Work out the finished part from the listing and answer in its coordinate system (mm). A direction names the side the tool comes from. Coordinates: 2 decimals unless noted, no trailing zeros. Order: outer loops, then holes, each group sorted by start corner. A loop starts at its lowest first (then second) coordinate and runs counter-clockwise, first axis right, second up. Notation, with made-up numbers: M -12.75,-29 L 46.25,-29 A17 cw 46.25,-15 Z; hole C 71.25,34.25 d8. An arc over 180 degrees is marked long. Write item = value, one per line. Start each with the question number.
Q1. Find section A-A on z = 18. Give the vertices of the cut face in (x, y), and give its area (3 significant figures).
Q2. Determine the mould class of faces 1 (the flat face through (5.735, -30.088, 12.325)), 2 (the flat face through (-5.735, 30.088, 12.325)), 3 (the flat face through (7.244, 27.181, 13.592)), 4 (the flat face through (0, 0, 0)) for opening direction X: released by +X, released by -X, zero draft, split by the parting line, or undercut.
Q3. Find section C-C on x = -27. Give the vertices of the cut face in (y, z), and give its area (3 significant figures).
Q4. Find section B-B on x = -10. Give the vertices of the cut face in (y, z), and give its area (3 significant figures).
Q5. Straight lines are drawn through the part: line 1 along Z through (x, y) = (-7, -9); line 2 along Y through (x, z) = (-26, 11.5); line 3 along Y through (x, z) = (16, 8.5). For each, find the intervals that lie inside material, in ascending order.
Q6. A tool of negligible diameter and unlimited length cuts with its end or side. For faces 5 (the flat face through (0, 0, 2.5)), 6 (the flat face through (27.1, -14.276, 12.325)), from which of +Z, -Z, +X, -X, +Y, -Y can it reach the whole face along a straight path? Write none if from no direction.
Q7. Each of these flat-tipped pins is pushed along its axis until it touches: P1, Ø4, axis at y = 14, z = 15.5, coming from the +X side; P2, Ø2, axis at x = 6.5, y = -10.5, coming from the +Z side; P3, Ø10, axis at y = -20.5, z = 3.5, coming from the -X side. Where does it stop, or does it pass through?
```python
from build123d import *

# Parameters (mm, degrees)
F1_DEPTH = 25
F2_T     = -2.5


with BuildPart() as f1:
    # F0 (on Top) → F1 (new body)
    with BuildSketch(Plane.XY):
        Polygon((-12.694525, 28.738617), (-23.90659, 20.384651), (-30.383662, 7.993256), (-30.842877, -5.981303), (-25.193282, -18.77119), (-14.553849, -27.843214), (-1.031847, -31.400547), (12.694525, -28.738617), (23.90659, -20.384651), (30.383662, -7.993256), (30.842877, 5.981303), (25.193282, 18.77119), (14.553849, 27.843214), (1.031847, 31.400547), align=None)
    extrude(amount=F1_DEPTH)

    # F2
    f2_openings = [f1.faces().sort_by_distance(p)[0] for p in [
        (0, 0, 25),
    ]]
    offset(amount=F2_T, openings=f2_openings)


solid = f1.part
```
Findings below:
q1.outline = M -30.84,-5.98 L -25.19,-18.77 L -14.55,-27.84 L -1.03,-31.4 L 12.69,-28.74 L 23.91,-20.38 L 30.38,-7.99 L 30.84,5.98 L 25.19,18.77 L 14.55,27.84 L 1.03,31.4 L -12.69,28.74 L -23.91,20.38 L -30.38,7.99 Z; hole M -28.33,-5.49 L -23.14,-17.24 L -13.37,-25.57 L -0.95,-28.84 L 11.66,-26.39 L 21.96,-18.72 L 27.9,-7.34 L 28.33,5.49 L 23.14,17.24 L 13.37,25.57 L 0.95,28.84 L -11.66,26.39 L -21.96,18.72 L -27.9,7.34 Z
q1.area = 469 mm^2
q2.face_1 = released by +X
q2.face_2 = released by -X
q2.face_3 = undercut
q2.face_4 = zero draft
q3.outline = M -14.68,0 L 14.47,0 L 14.47,25 L 9.07,25 L 9.07,2.5 L -8.49,2.5 L -8.49,25 L -14.68,25 Z
q3.area = 334 mm^2
q4.outline = M -29.04,0 L 29.26,0 L 29.26,25 L 26.71,25 L 26.71,2.5 L -26.46,2.5 L -26.46,25 L -29.04,25 Z
q4.area = 261 mm^2
q5.line_1 = 0 to 2.5
q5.line_2 = -16.94 to -10.76, 10.98 to 16.38
q5.line_3 = -26.28 to -23.16, 23.32 to 26.61
q6.face_5 = +Z
q6.face_6 = +Z, -Z, +X, -Y
q7.P1 = 28.18
q7.P2 = 2.5
q7.P3 = -26.64
